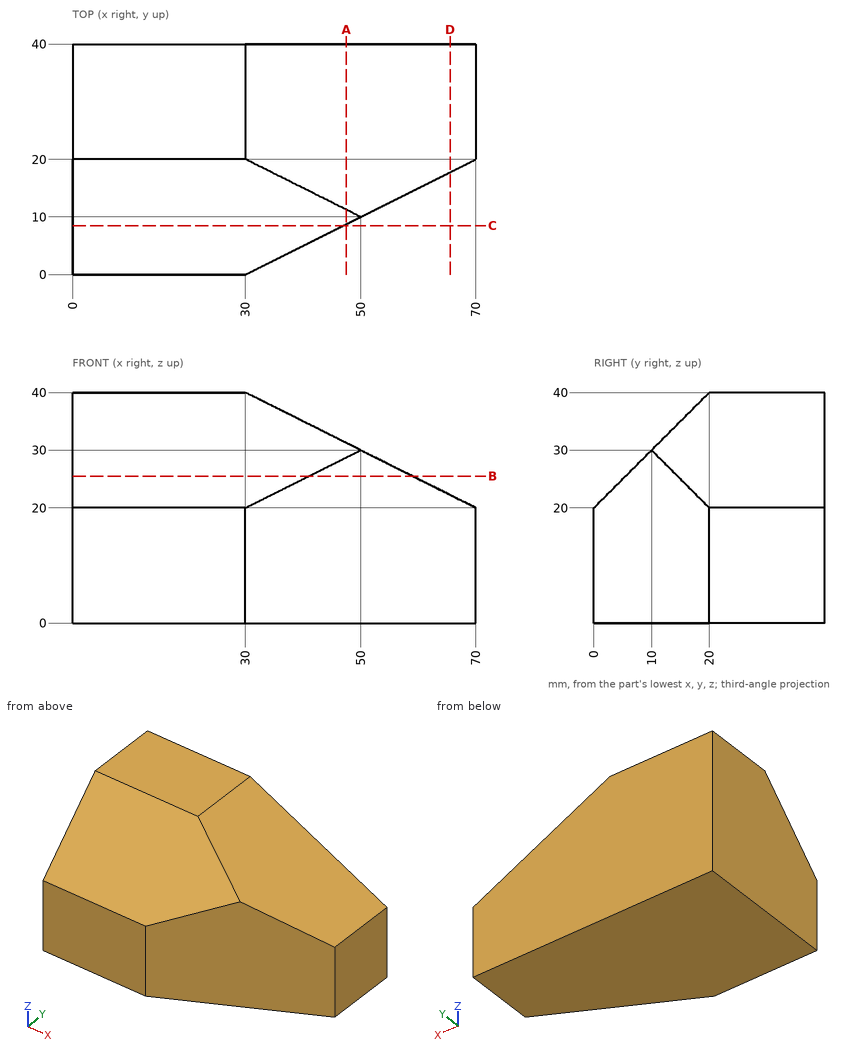
For this review, use the dimensioned drawing (mm, ordinates from the lowest corner) and the shaded views. Give positions to 0.01 mm unless a question says otherwise; leave off trailing zeros. Loops run counter-clockwise (first coordinate to the right, second up) from the corner with the lowest first, then second, coordinate; pieces in that order, holes last. Notation, with made-up numbers: (65, 81.25) -> (96, 81.25) arc R20 ccw to (96, 100.25) -> close; hole circle Ø11 at (18.25, 55.5). An arc over 180 degrees is marked (long way). Use CSV: the item, a comma, the result in double quotes.
1. Consider section C-C, the plane y = 8.5. Write out the cut boundary in (x, z), then the cut area to 3 significant figures.
Result:
outline,"(0, 0) -> (47, 0) -> (47, 28.5) -> (0, 28.5) -> close"
area,"1,340 mm²"
2. For P1, Ø6, axis at y = 11, z = 11.5, coming from the +X side; P2, Ø2, axis at x = 39.5, z = 31, coming from the -Y side, all flat-tipped, find the tip position at first contact; note any pin that passes through.
Result:
P1,"stops at x = 58"
P2,"stops at y = 10"
3. Consider section B-B, the plane z = 25.5. Write out the cut boundary in (x, y), then the cut area to 3 significant figures.
Result:
outline,"(0, 5.5) -> (41, 5.5) -> (59, 14.5) -> (59, 40) -> (0, 40) -> close"
area,"1,950 mm²"
4. To check wall thickness, follow probe 1 along X at (y, z) = (29.5, 30); probe 2 along Z at (x, y) = (39, 10); probe 3 along Y at (x, z) = (21.5, 37.5). State the ranges of each line that lie inside material, in increasing order. Write a range as from..to.
Result:
probe 1,"x = 0..50"
probe 2,"z = 0..30"
probe 3,"y = 17.5..40"
5. Consider section A-A, the plane x = 47.5. Write out the cut boundary in (y, z), then the cut area to 3 significant figures.
Result:
outline,"(8.75, 0) -> (40, 0) -> (40, 31.25) -> (11.25, 31.25) -> (8.75, 28.75) -> close"
area,"973 mm²"
6. Consider section D-D, the plane x = 65.5. Write out the cut boundary in (y, z), then the cut area to 3 significant figures.
Result:
outline,"(17.75, 0) -> (40, 0) -> (40, 22.25) -> (17.75, 22.25) -> close"
area,"495 mm²"
